The listing builds one solid part. Answer for the finished solid, in the listing's coordinates (mm). Coordinates: 2 decimals unless noted, no trailing zeros. Order: outer loops, then holes, each group sorted by start corner. A loop starts at its lowest first (then second) coordinate and runs counter-clockwise, first axis right, second up. Notation, with made-up numbers: M 45,39 L 89,39 A22 cw 89,56 Z; hole C 62.25,25.25 d9. An arc over 180 degrees is marked long. One line per item, written item: value. Start each with the question number.
Q1. The part is cut by section A-A on x = 7. Give the vertices of the cut face in (y, z), then the cut area to 3 significant figures.
Q2. The part is cut by section B-B on y = -2. Give the vertices of the cut face in (x, z), then the cut area to 3 significant figures.
Q3. A straight line is drawn through the part: line 1 along Z through (x, y) = (0, -2.5). Find the intervals that lie inside material, in ascending order. Write a range as [from, to].
```python
from build123d import *

# Parameters (mm, degrees)
SKETCH_W     = 37
SKETCH_H     = 24
PAD_DEPTH    = 15
SKETCH002_R  = 0.3
PAD001_DEPTH = 4.5
FILLET_R     = 0.3
FILLET001_R  = 0.3


with BuildPart() as part:
    # Sketch → Pad (new body)
    with BuildSketch(Plane.XY):
        Rectangle(SKETCH_W, SKETCH_H)
    extrude(amount=PAD_DEPTH)

    # Sketch002 (on Face5 of Pad) → Pad001 (join)
    with BuildSketch(Plane(origin=(0, 0, 0), x_dir=(1, 0, 0), z_dir=(0, 0, -1))):
        with Locations((-15.24, 8.89)):
            Circle(SKETCH002_R)
        with Locations((-10.16, 8.89)):
            Circle(SKETCH002_R)
        with Locations((10.16, -8.89)):
            Circle(SKETCH002_R)
        with Locations((15.24, -8.89)):
            Circle(SKETCH002_R)
        with Locations((-15.24, -8.89)):
            Circle(SKETCH002_R)
    extrude(amount=PAD001_DEPTH)

    # Fillet
    fillet_edges = [part.edges().sort_by_distance(p)[0] for p in [
        (18.5, -12, 7.5),
        (0, -12, 15),
        (-18.5, -12, 7.5),
        (-18.5, 0, 15),
        (-18.5, 12, 7.5),
        (18.5, 0, 15),
        (0, 12, 15),
        (18.5, 12, 7.5),
    ]]
    fillet(fillet_edges, radius=FILLET_R)

    # Fillet001
    fillet001_edges = [part.edges().sort_by_distance(p)[0] for p in [
        (14.94, 8.89, -4.5),
        (9.86, 8.89, -4.5),
        (-15.54, 8.89, -4.5),
        (-15.54, -8.89, -4.5),
        (-10.46, -8.89, -4.5),
    ]]
    fillet(fillet001_edges, radius=FILLET001_R)


solid = part.part
```
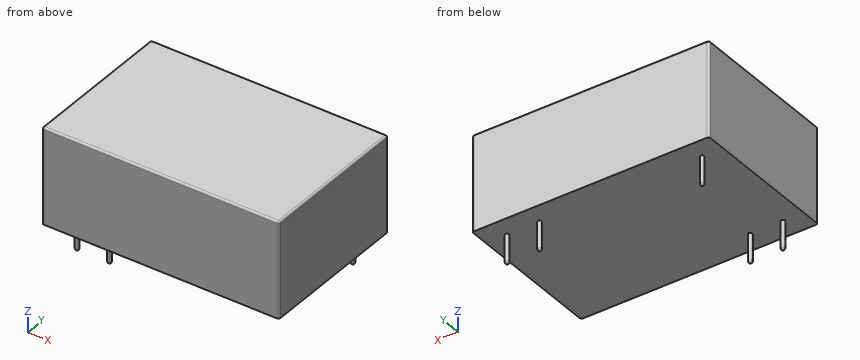
Output:
1. outline: M -12,0 L 12,0 L 12,14.7 A0.3 ccw 11.7,15 L -11.7,15 A0.3 ccw -12,14.7 Z
1. area: 360 mm^2
2. outline: M -18.5,0 L 18.5,0 L 18.5,14.7 A0.3 ccw 18.2,15 L -18.2,15 A0.3 ccw -18.5,14.7 Z
2. area: 555 mm^2
3. line 1: z = [0, 15]
